Can you work these out from the drawing? Everything is in mm from the part's minimum corner. Coordinates: 2 decimals unless noted, no trailing zeros. Loops run counter-clockwise (first coordinate to the right, second up) from the corner with the lowest first, then second, coordinate; pieces in that order, holes last. Notation, with made-up numbers: (-37.5, 20.25) -> (4.5, 20.25) arc R21 ccw to (4.5, 41.25) -> close; hole circle Ø5 at (47.5, 84). An arc over 180 degrees is marked (long way). Use one line per item in the form item = value. Start each with the question number.
(1) Imagine slicing it at A-A (x = 77.5). List the corners of the cut face in (y, z) for me.
(2) I'm going to push a flat-ended pin straight in: pin 1 (4 mm diameter, centred on x = 12.5, y = 77.5, fed in from -Z). Where does the tip first touch, or does it pass through?
(3) Imagine slicing it at B-B (y = 45). List the corners of the cut face in (x, z) for me.
(4) I need wall thicknesses on line 1 (Y direction, x = 77.5, z = 2.4); line 2 (X direction, y = 15, z = 4.55) (1 decimal). Which ranges of each line are inside material? Lowest first, please. Write a range as [from, to].
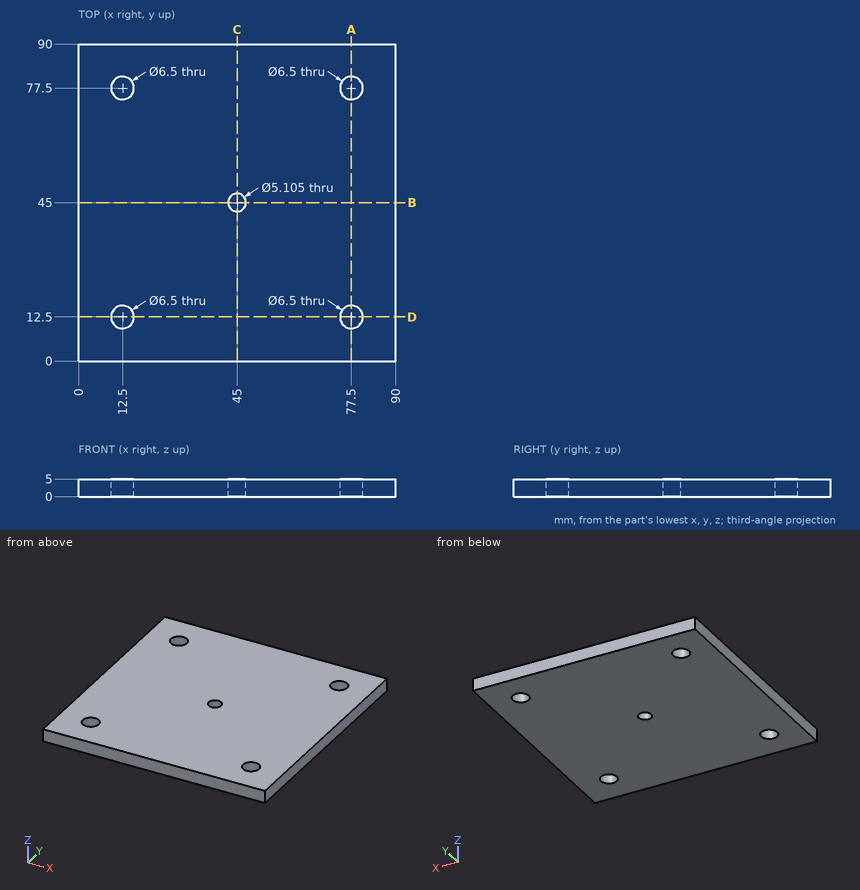
Worked out:
q1.outline = (0, 0) -> (9.25, 0) -> (9.25, 5) -> (0, 5) -> close; (15.75, 0) -> (74.25, 0) -> (74.25, 5) -> (15.75, 5) -> close; (80.75, 0) -> (90, 0) -> (90, 5) -> (80.75, 5) -> close
q2.pin_1 = through
q3.outline = (0, 0) -> (42.45, 0) -> (42.45, 5) -> (0, 5) -> close; (47.55, 0) -> (90, 0) -> (90, 5) -> (47.55, 5) -> close
q4.line_1 = [0, 9.25], [15.75, 74.25], [80.75, 90]
q4.line_2 = [0, 10.4], [14.6, 75.4], [79.6, 90]
